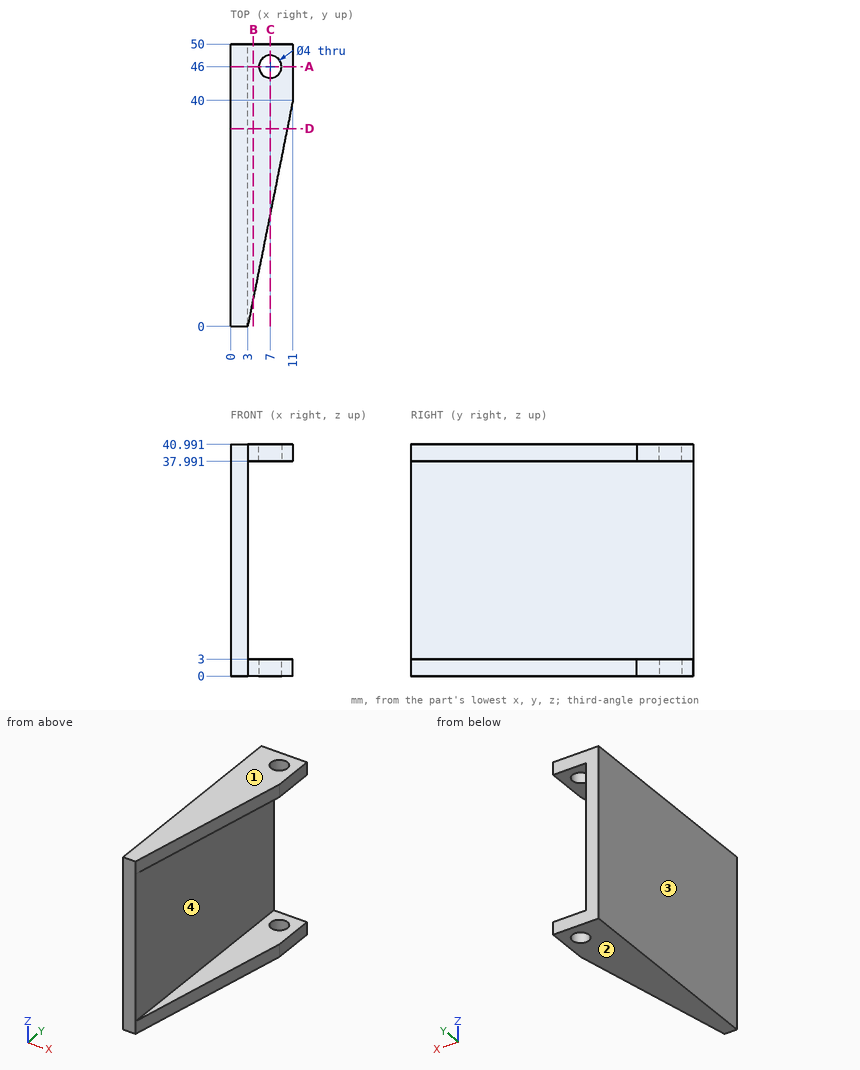
The figure shows three views and two pictorial views of one solid part (mm, origin at its lowest corner). Answer the questions. Coordinates: 2 decimals unless noted, no trailing zeros. Loops run counter-clockwise (first coordinate to the right, second up) from the corner with the lowest first, then second, coordinate; pieces in that order, holes last.
1) Find section D-D on y = 35. Write down the section's boundary in (x, z), then the cut area to 3 significant figures.
2) Find section B-B on x = 4. Write down the section's boundary in (y, z).
3) Find the intervals of material crossed by L1, parallel to Z at x = 4.75, y = 32.5; L2, parallel to X at y = 15.5, z = 16; L3, parallel to X at y = 10.5, z = 2, in increasing order.
4) Find section A-A on y = 46. Write down the section's boundary in (x, z), then the cut area to 3 significant figures.
5) Determine the mould class of the marked faces 1, 2, 3 and 4 for opening direction Z: pulls with the +Z half, pulls with the -Z half, needs draft (parallel to the pull), parting line crosses it, or undercut.
6) Find section C-C on x = 7. Write down the section's boundary in (y, z), then the cut area to 3 significant figures.
7) A flat-ended cylindrical pin translates along its axis: pin 1 Ø5 at (y, z) = (9.5, 21) entering from +X. Find the tip coordinate at first contact, or state that the pin passes through.
Values:
1. outline: (0, 0) - (10, 0) - (10, 3) - (3, 3) - (3, 37.99) - (10, 37.99) - (10, 40.99) - (0, 40.99) - close
1. area: 165 mm2
2. outline: (5, 0) - (50, 0) - (50, 3) - (5, 3) - close; (5, 37.99) - (50, 37.99) - (50, 40.99) - (5, 40.99) - close
3. L1: z = 0 to 3, 37.99 to 40.99
3. L2: x = 0 to 3
3. L3: x = 0 to 5.1
4. outline: (0, 0) - (5, 0) - (5, 3) - (3, 3) - (3, 37.99) - (5, 37.99) - (5, 40.99) - (0, 40.99) - close; (9, 0) - (11, 0) - (11, 3) - (9, 3) - close; (9, 37.99) - (11, 37.99) - (11, 40.99) - (9, 40.99) - close
4. area: 147 mm2
5. face 1: pulls with the +Z half
5. face 2: pulls with the -Z half
5. face 3: needs draft
5. face 4: undercut
6. outline: (20, 0) - (44, 0) - (44, 3) - (20, 3) - close; (20, 37.99) - (44, 37.99) - (44, 40.99) - (20, 40.99) - close; (48, 0) - (50, 0) - (50, 3) - (48, 3) - close; (48, 37.99) - (50, 37.99) - (50, 40.99) - (48, 40.99) - close
6. area: 156 mm2
7. pin 1: stops at x = 3
